The listing builds one solid part. Answer for the finished solid, in the listing's coordinates (mm). A direction names the side the tool comes from. Give positions to 0.01 mm unless a question says otherwise; leave off trailing zeros. Order: outer loops, then holes, each group sorted by start corner. A loop starts at its lowest first (then second) coordinate and runs counter-clockwise, first axis right, second up. Notation, with made-up numbers: (-22.75, -33) - (33.25, -33) arc R18 ccw to (33.25, -26) - close; hole circle Ø5 at (-37.5, 79). An arc over 180 degrees is marked (long way). Write each question's results on one line, items separated by ' | '. Start each with the question number.
1. Determine the mould class of faces 3 (the face through (0, -0.2, -54.7)), 4 (the face through (45.308, -0.304, -81.758)), 5 (the face through (69, 10, -110.6)) for opening direction X: released by +X, released by -X, zero draft, split by the parting line, or undercut.
2. Which of the six approach directions +Z, -Z, +X, -X, +Y, -Y give full straight-line access (tool end or side, diameter ignored) to faces 1 (the face through (69, 0, -54)), 2 (the face through (69, 10, 0.6))?
3. Section A-A (y = 1.5) is taken. Give the vertices of the cut face in (x, z).
4. A flat-ended cylindrical pin translates along its axis: pin 1 (5 mm diameter, centred on x = 43.65, z = -80.24, fed in from +Y). Find the tip coordinate at first contact, or state that the pin passes through.
5. Section C-C (x = 24) is taken. Give the vertices of the cut face in (y, z).
6. Find the intervals of material crossed by L1, parallel to Z at x = 43.65, y = -0.35; L2, parallel to Z at x = 71.5, y = 17.25; L3, parallel to Y at x = 40, z = -64, in increasing order.
7. Section B-B (x = 43.65) is taken. Give the vertices of the cut face in (y, z), and give its area (3 significant figures).
8. Section D-D (z = -16) is taken. Give the vertices of the cut face in (x, y), and give its area (3 significant figures).
from build123d import *

# Parameters (mm, degrees)
CROQUIS1_W                   = 110
CROQUIS1_H                   = 20
SALIENTE_EXTRUIR1_DEPTH      = 140
VACIADO1_T                   = 0.6
TALADRO_DE_MARGEN_PARA_M42_D = 4.5


with BuildPart() as part:
    # Croquis1 → Saliente-Extruir1 (new body)
    with BuildSketch(Plane(origin=(0, 0, 0), x_dir=(0, 0, -1), z_dir=(1, 0, 0))):
        with Locations((55, 10)):
            Rectangle(CROQUIS1_W, CROQUIS1_H)
    extrude(amount=SALIENTE_EXTRUIR1_DEPTH)

    # Vaciado1
    vaciado1_openings = [part.faces().sort_by_distance(p)[0] for p in [
        (70, 20, -55),
        (0, 10, -55),
        (140, 10, -55),
    ]]
    offset(amount=VACIADO1_T, openings=vaciado1_openings, kind=Kind.INTERSECTION)

    # Taladro de margen para M42 (through all)
    with Locations(Plane(origin=(104.234059149, 1, -171.2), x_dir=(1, 0, 0), z_dir=(0, 1, 0))):
        with Locations((-60.584059149, -90.9625), (-60.584059149, -106.8375), (-60.584059149, -125.5625), (-60.584059149, -141.4375)):
            Hole(TALADRO_DE_MARGEN_PARA_M42_D / 2)


solid = part.part
Reported:
1) face 3: released by -X | face 4: undercut | face 5: zero draft
2) face 1: +X, -X, +Y | face 2: +Z, +X, -X, +Y, -Y
3) outline: (0, -110.6) - (140, -110.6) - (140, -110) - (0, -110) - close; (0, 0) - (140, 0) - (140, 0.6) - (0, 0.6) - close
4) pin 1: y = 0
5) outline: (-0.6, -110.6) - (20, -110.6) - (20, -110) - (0, -110) - (0, 0) - (20, 0) - (20, 0.6) - (-0.6, 0.6) - close
6) L1: -110.6 to -82.49, -77.99 to -66.61, -62.11 to -47.89, -43.39 to -32.01, -27.51 to 0.6 | L2: -110.6 to -110, 0 to 0.6 | L3: -0.6 to 0
7) outline: (-0.6, -110.6) - (20, -110.6) - (20, -110) - (0, -110) - (0, -82.49) - (-0.6, -82.49) - close; (-0.6, -77.99) - (0, -77.99) - (0, -66.61) - (-0.6, -66.61) - close; (-0.6, -62.11) - (0, -62.11) - (0, -47.89) - (-0.6, -47.89) - close; (-0.6, -43.39) - (0, -43.39) - (0, -32.01) - (-0.6, -32.01) - close; (-0.6, -27.51) - (0, -27.51) - (0, 0) - (20, 0) - (20, 0.6) - (-0.6, 0.6) - close | area: 79.9 mm²
8) outline: (0, -0.6) - (140, -0.6) - (140, 0) - (0, 0) - close | area: 84.0 mm²
